from build123d import *

# Parameters (mm, degrees)
SKETCH1_W           = 16.6
SKETCH1_H           = 8
BOSS_EXTRUDE1_DEPTH = 2
SKETCH2_R           = 2.5
SKETCH2_R_2         = 1.5
BOSS_EXTRUDE2_DEPTH = 4
SKETCH3_W           = 16.6
SKETCH3_H           = 2
BOSS_EXTRUDE3_DEPTH = 8


with BuildPart() as part:
    # Sketch1 → Boss-Extrude1 (new body)
    with BuildSketch(Plane(origin=(0, 0, 0), x_dir=(1, 0, 0), z_dir=(0, 1, 0))):
        Rectangle(SKETCH1_W, SKETCH1_H)
    extrude(amount=BOSS_EXTRUDE1_DEPTH)

    # Sketch2 → Boss-Extrude2 (add)
    with BuildSketch(Plane(origin=(0, 2, 0), x_dir=(1, 0, 0), z_dir=(0, 1, 0))):
        with Locations(Location((-3.25, 0, 0), (0, 0, 90))):
            Circle(SKETCH2_R)
        with Locations(Location((3.25, 0, 0), (0, 0, 90))):
            Circle(SKETCH2_R_2)
    extrude(amount=BOSS_EXTRUDE2_DEPTH)

    # Sketch3 → Boss-Extrude3 (add)
    with BuildSketch(Plane.XZ):
        with Locations((0, -3)):
            Rectangle(SKETCH3_W, SKETCH3_H)
    extrude(amount=BOSS_EXTRUDE3_DEPTH)


solid = part.part
Input: part model. Units: mm. Frame: model coordinates. A direction names the side the tool comes from. Coordinates: 2 decimals unless noted, no trailing zeros. Order: outer loops, then holes, each group sorted by start corner. A loop starts at its lowest first (then second) coordinate and runs counter-clockwise, first axis right, second up. Notation, with made-up numbers: M -35.75,-3 L -3.75,-3 A27 ccw -3.75,19 Z; hole C -1.75,77.5 d4. An arc over 180 degrees is marked long. One line per question, with ' | ' between items.
Item 1: Reachability of faces 4 (the flat face through (-3, 6, 0)), 5 (the cylindrical face through (1.763, 3.972, 0.195)), 6 (the flat face through (0, 0, 1)) from +Z, -Z, +X, -X, +Y, -Y: full face, straight path, thin tool, end or side. Return the list, or none.
Geometry results:
face 4: +Z, -Z, +X, -X, +Y | face 5: +Y | face 6: +Z, +X, -X, -Y
Item 2: Section D-D (x = 3.25). Output: boundary loops of the cut face in (y, z), then the cut area to 3 significant figures.
Geometry results:
outline: M -8,-4 L 2,-4 L 2,-1.5 L 6,-1.5 L 6,1.5 L 2,1.5 L 2,4 L 0,4 L 0,-2 L -8,-2 Z | area: 44.0 mm^2
Item 3: Section A-A (z = 0). Output: boundary loops of the cut face in (x, y), then the cut area to 3 significant figures.
Geometry results:
outline: M -8.3,0 L 8.3,0 L 8.3,2 L 4.75,2 L 4.75,6 L 1.75,6 L 1.75,2 L -0.75,2 L -0.75,6 L -5.75,6 L -5.75,2 L -8.3,2 Z | area: 65.2 mm^2
Item 4: Pin query (flat end, axial travel): pin 1 (1.8 mm diameter, centred on x = 3.5, z = 1, fed in from -Y). Return the tip coordinate at first contact, or that it passes through.
Geometry results:
pin 1: stops at y = 0
Item 5: Section B-B (x = -3.25). Output: boundary loops of the cut face in (y, z).
Geometry results:
outline: M -8,-4 L 2,-4 L 2,-2.5 L 6,-2.5 L 6,2.5 L 2,2.5 L 2,4 L 0,4 L 0,-2 L -8,-2 Z
Item 6: Ray query, line 1 along Y through (x, z) = (-3.5, -3); line 2 along Z through (x, y) = (2, -4.5); line 3 along X through (y, z) = (3.5, 0.25). Return the intervals inside material, ascending.
Geometry results:
line 1: y = -8 to 2 | line 2: z = -4 to -2 | line 3: x = -5.74 to -0.76, 1.77 to 4.73
Item 7: Section C-C (y = 2.5). Output: boundary loops of the cut face in (x, z).
Geometry results:
outline: C -3.25,0 d5; C 3.25,0 d3
Item 8: Draft query along X for faces 1 (the flat face through (0, -4, -2)), 2 (the flat face through (8.3, -1, -3)), 3 (the cylindrical face through (-1.729, 3.972, 1.984)). Return one class per face: released by +X, released by -X, zero draft, split by the parting line, or undercut.
Geometry results:
face 1: zero draft | face 2: released by +X | face 3: undercut
